Can you work these out from the drawing? Everything is in mm from the part's minimum corner. A direction names the side the tool comes from. Coordinates: 2 decimals unless noted, no trailing zeros. Loops run counter-clockwise (first coordinate to the right, second up) from the corner with the lowest first, then second, coordinate; pieces in that order, holes last.
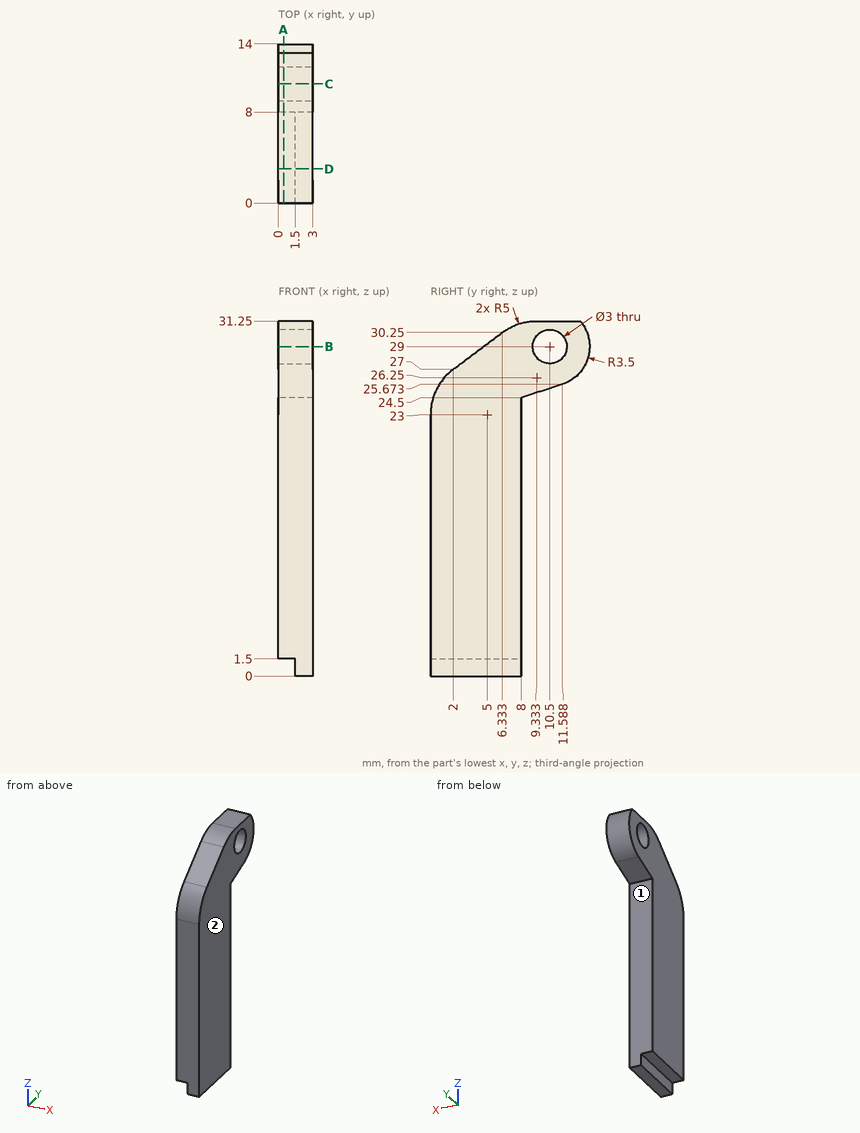
1) Imagine slicing it at D-D on y = 3. List the corners of the cut face in (x, z) for me, plus the area to 3 significant figures.
2) Imagine slicing it at A-A on x = 0.45. List the corners of the cut face in (y, z) for me.
3) Will these pins go through, and if not, where does the flat tip stop? pin 1 (1 mm diameter, centred on x = 2.5, y = 7.5, fed in from +Z); pin 2 (1.2 mm diameter, centred on y = 5.5, z = 0.5, fed in from -X); pin 3 (0.8 mm diameter, centred on x = 0.5, y = 2.5, fed in from -Z).
4) Imagine slicing it at B-B on z = 29. List the corners of the cut face in (x, y) for me.
5) If I drill on L1, parallel to Y at x = 2.5, z = 9; L2, parallel to Z at x = 0.8, y = 10.5; L3, parallel to Y at x = 1.75, z = 29 (1 decimal), over which ranges is the centre line in solid material (lowest first)?
6) Imagine slicing it at C-C on y = 10.5. List the corners of the cut face in (x, z) for me.
7) For the marked faces 1 and 2, which set-ups out of +Z, -Z, +X, -X, +Y, -Y let a thin tool reach every point of the face, with its end or its side?
Solved:
1. outline: (0, 1.5) - (1.5, 1.5) - (1.5, 0) - (3, 0) - (3, 27.75) - (0, 27.75) - close
1. area: 81.0 mm2
2. outline: (0, 1.5) - (8, 1.5) - (8, 24.5) - (11.59, 25.67) arc R3.5 ccw to (13.18, 31.25) - (9.33, 31.25) arc R5 ccw to (6.33, 30.25) - (2, 27) arc R5 ccw to (0, 23) - close; hole circle Ø3 at (10.5, 29)
3. pin 1: stops at z = 31.07
3. pin 2: stops at x = 1.5
3. pin 3: stops at z = 1.5
4. outline: (0, 4.67) - (3, 4.67) - (3, 9) - (0, 9) - close; (0, 12) - (3, 12) - (3, 14) - (0, 14) - close
5. L1: y = 0 to 8
5. L2: z = 25.32 to 27.5, 30.5 to 31.25
5. L3: y = 4.7 to 9, 12 to 14
6. outline: (0, 25.32) - (3, 25.32) - (3, 27.5) - (0, 27.5) - close; (0, 30.5) - (3, 30.5) - (3, 31.25) - (0, 31.25) - close
7. face 1: -Z, +X, -X, +Y
7. face 2: +Z, -Z, +X, +Y, -Y
